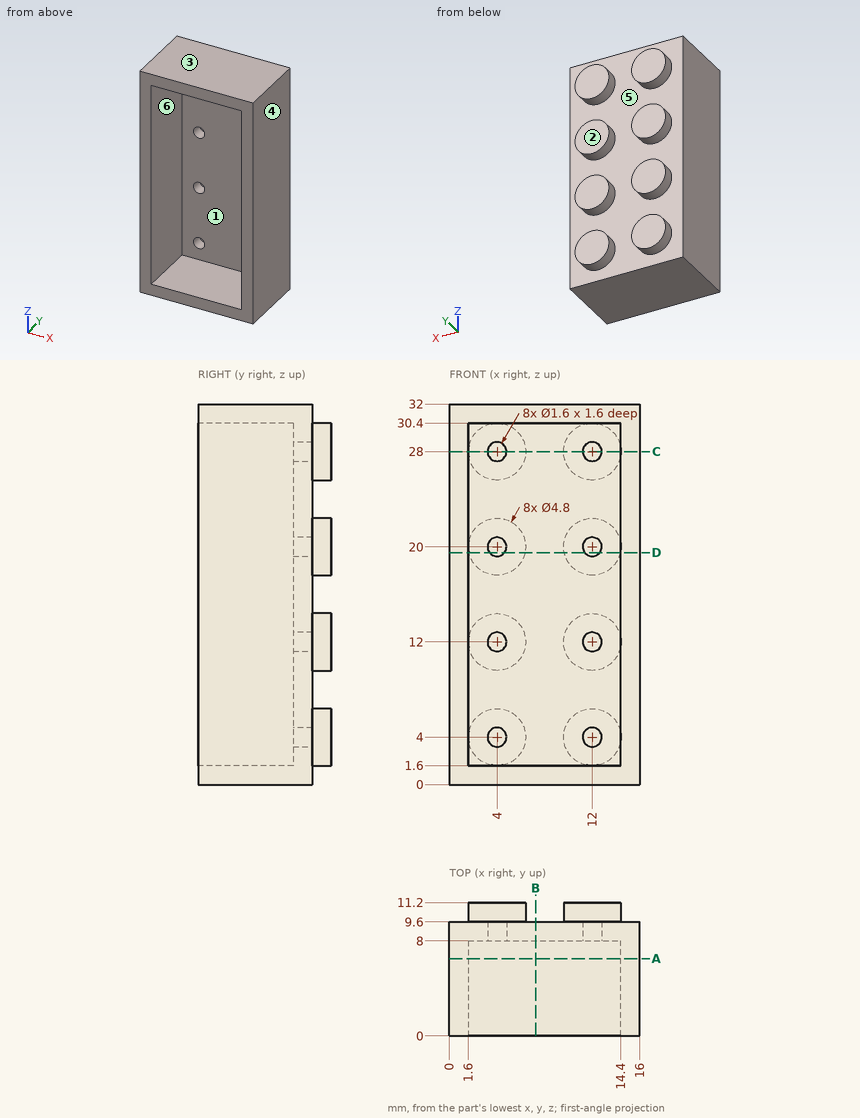
For this review, use the dimensioned drawing (mm, ordinates from the lowest corner) and the shaded views. A direction names the side the tool comes from. Give positions to 0.01 mm unless a question says otherwise; leave off trailing zeros. Loops run counter-clockwise (first coordinate to the right, second up) from the corner with the lowest first, then second, coordinate; pieces in that order, holes last. Notation, with made-up numbers: (37.25, 15.5) -> (83.25, 15.5) arc R21 ccw to (83.25, 38.5) -> close; hole circle Ø6 at (30, -3.5). An arc over 180 degrees is marked (long way). One line per question, with ' | ' between items. Start each with the question number.
(1) For the marked faces 4, 5 and 6, list the 3-axis set-ups (+Z, -Z, +X, -X, +Y, -Y) from which the entire face can be reached by the end or side of a thin tool; tool diameter is ignored.
(2) We need section A-A (y = 6.5). State the section outline as (x, z) points, and give its area (3 significant figures).
(3) Insertion check: P1, Ø2, axis at x = 10, z = 27, coming from the -Y side; P2, Ø1.5, axis at x = 4.5, y = 6.5, coming from the -Z side; P3, Ø0.5, axis at x = 12, z = 12, coming from the -Y side. Each pin has a flat end and moves straight along its axis. Give the tip position at first contact, or say it passes through.
(4) For line 1 (Z direction, x = 4, y = 10); line 2 (X direction, y = 8.85, z = 28); line 3 (X direction, y = 3, z = 26), list the stretches that pass through material, from the lowest coordinate up.
(5) We need section B-B (x = 7.25). State the section outline as (y, z) points, and give its area (3 significant figures).
(6) Draft analysis for pull direction Z (two halves, no side actions). For the marked faces 1, 2 and 3, state which applies: +Z half, -Z half, draft (parallel to the pull), parting line (faces both ways), or undercut.
(7) We need section C-C (z = 28). State the section outline as (x, y) points, and give its area (3 significant figures).
(8) We need section D-D (z = 19.5). State the section outline as (x, y) points, and give its area (3 significant figures).
The answers:
1) face 4: +Z, -Z, +X, +Y, -Y | face 5: +Y | face 6: -Y
2) outline: (0, 0) -> (16, 0) -> (16, 32) -> (0, 32) -> close; hole (1.6, 1.6) -> (14.4, 1.6) -> (14.4, 30.4) -> (1.6, 30.4) -> close | area: 143 mm^2
3) P1: stops at y = 8 | P2: stops at z = 0 | P3: stops at y = 9.6
4) line 1: z = 1.6 to 6.4, 9.6 to 14.4, 17.6 to 22.4, 25.6 to 30.4 | line 2: x = 0 to 3.2, 4.8 to 11.2, 12.8 to 16 | line 3: x = 0 to 1.6, 14.4 to 16
5) outline: (0, 0) -> (9.6, 0) -> (9.6, 32) -> (0, 32) -> (0, 30.4) -> (8, 30.4) -> (8, 1.6) -> (0, 1.6) -> close | area: 76.8 mm^2
6) face 1: undercut | face 2: draft | face 3: +Z half
7) outline: (0, 0) -> (1.6, 0) -> (1.6, 8) -> (3.2, 8) -> (3.2, 9.6) -> (4.8, 9.6) -> (4.8, 8) -> (11.2, 8) -> (11.2, 9.6) -> (12.8, 9.6) -> (12.8, 8) -> (14.4, 8) -> (14.4, 0) -> (16, 0) -> (16, 9.6) -> (14.4, 9.6) -> (14.4, 11.2) -> (9.6, 11.2) -> (9.6, 9.6) -> (6.4, 9.6) -> (6.4, 11.2) -> (1.6, 11.2) -> (1.6, 9.6) -> (0, 9.6) -> close | area: 61.4 mm^2
8) outline: (0, 0) -> (1.6, 0) -> (1.6, 8) -> (3.38, 8) -> (3.38, 9.6) -> (4.62, 9.6) -> (4.62, 8) -> (11.38, 8) -> (11.38, 9.6) -> (12.62, 9.6) -> (12.62, 8) -> (14.4, 8) -> (14.4, 0) -> (16, 0) -> (16, 9.6) -> (14.35, 9.6) -> (14.35, 11.2) -> (9.65, 11.2) -> (9.65, 9.6) -> (6.35, 9.6) -> (6.35, 11.2) -> (1.65, 11.2) -> (1.65, 9.6) -> (0, 9.6) -> close | area: 62.2 mm^2
